Here's how the part is built. I have some questions about the finished solid (model axes, mm). Face numbers are marked on the shaded views. A direction names the side the tool comes from. Give positions to 0.01 mm unless a question says otherwise; leave off trailing zeros. Write each loop counter-clockwise with the first axis right and the second up, starting at its lowest first coordinate (ties: lowest second). Pieces come first, ordered by that corner, then holes. Notation, with made-up numbers: (-33.5, 53.25) -> (-17.5, 53.25) arc R5 ccw to (-17.5, 57.25) -> close; hole circle Ø4 at (13.5, -26). An arc over 180 degrees is marked (long way). Use CSV: the item, a comma, the result in double quotes. Start each with the question number.
(1) Which directions (+Z, -Z, +X, -X, +Y, -Y) give clear straight access to the entire face, cutting with the end or side of a thin tool? Please do the marked faces 4, 5 and 6.
(2) Suppose I cut it at C-C on y = 17.5. List the corners of the cut face in (x, z) for me, plus the area to 3 significant figures.
(3) I need wall thicknesses on L1, parallel to Y at x = 0.45, z = 0.2; L2, parallel to Y at x = 1.75, z = 0.6; L3, parallel to Z at x = -0.3, y = 16.5. Which ranges of each line are inside material? Lowest first, please. Write a range as [from, to].
(4) Suppose I cut it at A-A on x = 0. List the corners of the cut face in (y, z) for me.
(5) If we mould it in two halves opening along X, with no side actions, what happens to the marked faces 1, 2 and 3? For each: pulls with the +X half, pulls with the -X half, needs draft (parallel to the pull), parting line crosses it, or undercut.
(6) Suppose I cut it at B-B on z = 0. List the corners of the cut face in (x, y) for me.
(7) For pin 1 Ø2 at (y, z) = (14.5, 0) entering from -X, with a flat end and sliding along its axis, tell me the tip position at first contact or that it passes through.
from build123d import *

# Parameters (mm, degrees)
SKETCH1_R             = 2.71
BOSS_EXTRUDE1_DEPTH   = 10
SKETCH2_OUTSIDE_W     = 9.94
SKETCH2_OUTSIDE_H     = 9.94
SKETCH2_OUTSIDE_R     = 1.5
CUT_EXTRUDE1_DEPTH    = 7.92
FILLET1_R             = 0.25
FILLET2_R             = 0.15
SKETCH3_W             = 1.2
SKETCH3_H             = 5.422046684
CUT_EXTRUDE2_DEPTH    = 0.9
BODY_MOVE_COPY1_ANGLE = 180


with BuildPart() as part:
    # Sketch1 → Boss-Extrude1 (new body)
    with BuildSketch(Plane(origin=(0, 0, 0), x_dir=(1, 0, 0), z_dir=(0, 1, 0))):
        with Locations(Location((0, 0, 0), (0, 0, 270))):
            Circle(SKETCH1_R)
    extrude(amount=BOSS_EXTRUDE1_DEPTH)

    # Sketch2 outside → Cut-Extrude1 (cut)
    with BuildSketch(Plane(origin=(0, 10, 0), x_dir=(1, 0, 0), z_dir=(0, 1, 0))):
        Rectangle(SKETCH2_OUTSIDE_W, SKETCH2_OUTSIDE_H)
        with Locations(Location((0, 0, 0), (0, 0, 270))):
            Circle(SKETCH2_OUTSIDE_R, mode=Mode.SUBTRACT)
    extrude(amount=-CUT_EXTRUDE1_DEPTH, mode=Mode.SUBTRACT)

    # Fillet1
    fillet1_edges = [part.edges().sort_by_distance(p)[0] for p in [
        (0, 0, -2.71),
        (0, 2.08, -2.71),
    ]]
    fillet(fillet1_edges, radius=FILLET1_R)

    # Fillet2
    fillet2_edges = [part.edges().sort_by_distance(p)[0] for p in [
        (0, 2.08, -1.5),
    ]]
    fillet(fillet2_edges, radius=FILLET2_R)

    # Sketch3 → Cut-Extrude2 (cut)
    with BuildSketch(Plane.XZ):
        Rectangle(SKETCH3_W, SKETCH3_H)
    extrude(amount=-CUT_EXTRUDE2_DEPTH, mode=Mode.SUBTRACT)


with BuildPart() as part_1:
    # Body-Move/Copy1: moved
    add(part.part.rotate(Axis((0, 10, 0), (1, 0, 0)), BODY_MOVE_COPY1_ANGLE))


solid = part_1.part
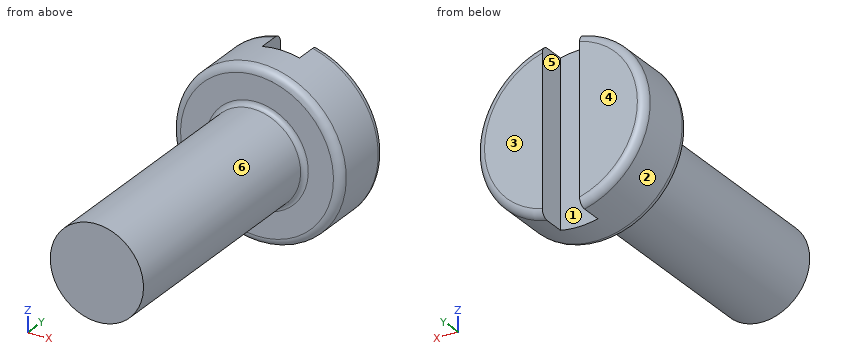
Geometry says:
1,face 4,"+Z, -Z, +X, -X, +Y"
1,face 5,"+Z, -Z, +Y"
1,face 6,"-Y"
2,outline,"circle Ø3 at (0, 0)"
2,area,"7.07 mm²"
3,L1,"[10, 19.1]"
3,L2,"[17.92, 20]"
3,L3,"[-1.47, 1.47]"
4,outline,"(10, -1.5) -> (17.77, -1.5) arc R0.15 cw to (17.92, -1.65) -> (17.92, -2.46) arc R0.25 ccw to (18.17, -2.71) -> (19.1, -2.71) -> (19.1, 2.71) -> (18.17, 2.71) arc R0.25 ccw to (17.92, 2.46) -> (17.92, 1.65) arc R0.15 cw to (17.77, 1.5) -> (10, 1.5) -> close"
5,face 1,"undercut"
5,face 2,"parting line crosses it"
5,face 3,"needs draft"
6,outline,"(-2.71, 18.17) arc R0.25 ccw to (-2.46, 17.92) -> (-1.65, 17.92) arc R0.15 cw to (-1.5, 17.77) -> (-1.5, 10) -> (1.5, 10) -> (1.5, 17.77) arc R0.15 cw to (1.65, 17.92) -> (2.46, 17.92) arc R0.25 ccw to (2.71, 18.17) -> (2.71, 19.75) arc R0.25 ccw to (2.46, 20) -> (0.6, 20) -> (0.6, 19.1) -> (-0.6, 19.1) -> (-0.6, 20) -> (-2.46, 20) arc R0.25 ccw to (-2.71, 19.75) -> close"
7,pin 1,"x = -1.5"
